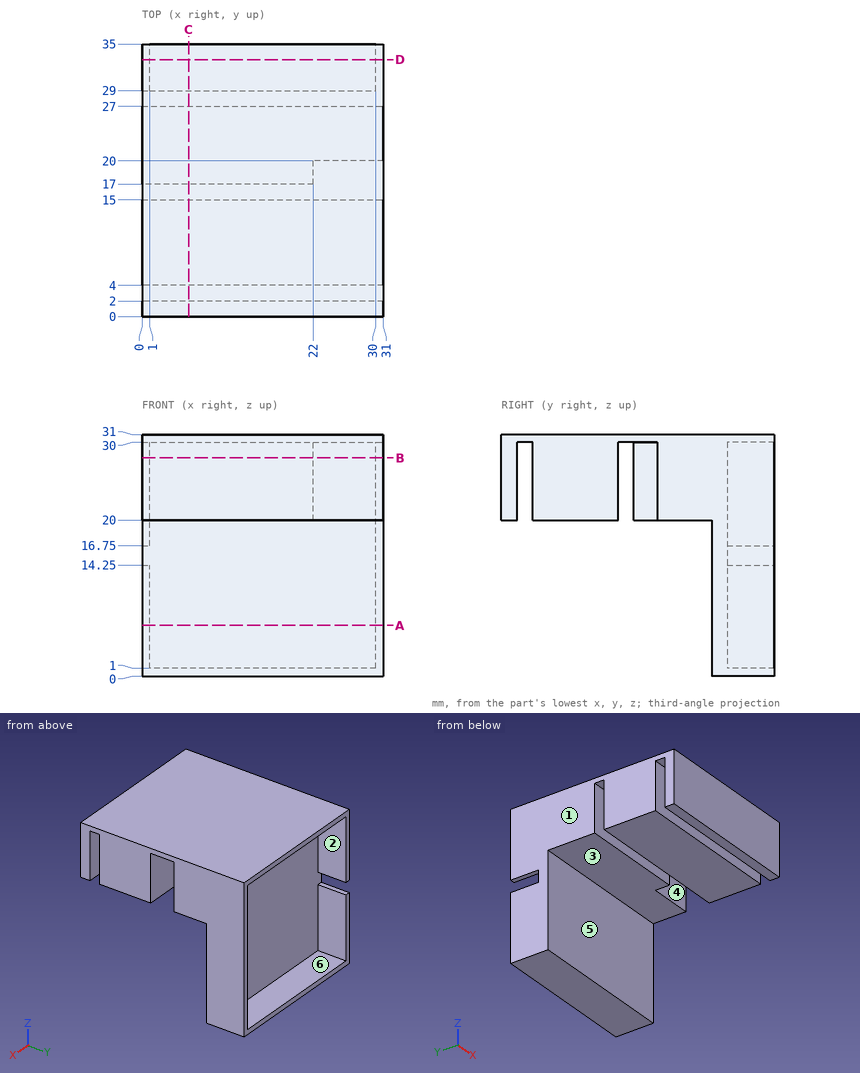
Part print with two shaded views. Sizes in mm from the minimum x, y, z corner. A direction names the side the tool comes from. Coordinates: 2 decimals unless noted, no trailing zeros. Write each loop counter-clockwise with the first axis right and the second up, starting at its lowest first coordinate (ties: lowest second). Pieces come first, ordered by that corner, then holes.
(1) Cut at B-B on z = 28. List the corners of the cut face in (x, y), and give its area (3 significant figures).
(2) 3-axis set-ups, long thin cutter, end or side, ignore diameter. For the marked faces 4, 5 and 6: which of +Z, -Z, +X, -X, +Y, -Y reach the whole face in a straight line?
(3) Cut at A-A on z = 6.5. List the corners of the cut face in (x, y).
(4) Mould opens along Z. For the marked faces 1, 2 and 3 say: pulls with the +Z half, pulls with the -Z half, needs draft (parallel to the pull), parting line crosses it, or undercut.
(5) Pin check, flat tips, straight feed: pin 1 Ø8 at (x, z) = (5.5, 14.5) entering from -Y; pin 2 Ø0.6 at (x, y) = (21, 3) entering from -Z; pin 3 Ø5.5 at (x, y) = (10, 11) entering from -Z. Stop position of each tip, or through.
(6) Cut at D-D on y = 33. List the corners of the cut face in (x, z), and give its area (4 significant figures).
(7) Drill centre lines: line 1 (Y direction, x = 2.5, z = 27); line 2 (Z direction, x = 7, y = 30); line 3 (Y direction, x = 24.5, z = 25). Where is each one in solid material? Low to high.
(8) Cut at C-C on x = 6. List the corners of the cut face in (y, z).
Working result:
1. outline: (0, 0) - (31, 0) - (31, 2) - (0, 2) - close; (0, 4) - (31, 4) - (31, 15) - (0, 15) - close; (0, 17) - (22, 17) - (22, 20) - (31, 20) - (31, 35) - (30, 35) - (30, 29) - (1, 29) - (1, 35) - (0, 35) - close
1. area: 760 mm2
2. face 4: -Z, +X
2. face 5: -Z, +X, -X, -Y
2. face 6: +Y
3. outline: (0, 27) - (31, 27) - (31, 35) - (30, 35) - (30, 29) - (1, 29) - (1, 35) - (0, 35) - close
4. face 1: needs draft
4. face 2: undercut
4. face 3: pulls with the -Z half
5. pin 1: stops at y = 27
5. pin 2: stops at z = 30
5. pin 3: stops at z = 20
6. outline: (0, 0) - (31, 0) - (31, 31) - (0, 31) - (0, 16.75) - (1, 16.75) - (1, 30) - (30, 30) - (30, 1) - (1, 1) - (1, 14.25) - (0, 14.25) - close
6. area: 117.5 mm2
7. line 1: y = 0 to 2, 4 to 15, 17 to 29
7. line 2: z = 0 to 1, 30 to 31
7. line 3: y = 0 to 2, 4 to 15, 20 to 29
8. outline: (0, 20) - (2, 20) - (2, 30) - (4, 30) - (4, 20) - (15, 20) - (15, 30) - (17, 30) - (17, 20) - (27, 20) - (27, 0) - (35, 0) - (35, 1) - (29, 1) - (29, 30) - (35, 30) - (35, 31) - (0, 31) - close
